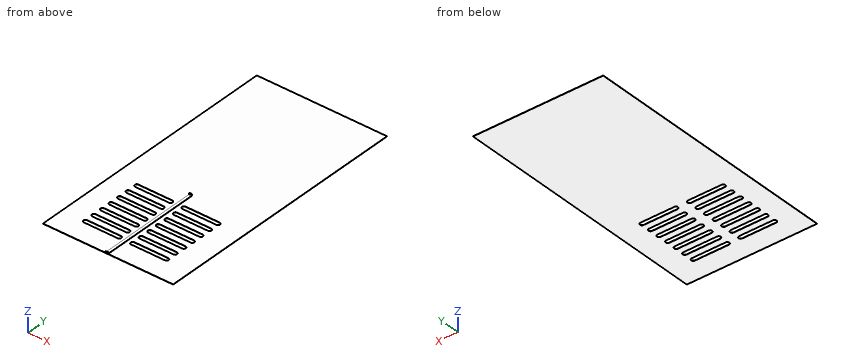
```python
from build123d import *

# Parameters (mm, degrees)
SKETCH1_W           = 500
SKETCH1_H           = 1000
BOSS_EXTRUDE1_DEPTH = 0.8
SKETCH4_W           = 10.782807929
SKETCH4_H           = 393.4
BOSS_EXTRUDE3_DEPTH = 0.8
SKETCH6_W           = 10.782807929
SKETCH6_H           = 5
BOSS_EXTRUDE4_DEPTH = 0.8
SKETCH7_W           = 10.782807929
SKETCH7_H           = 5
BOSS_EXTRUDE5_DEPTH = 0.8


with BuildPart() as part:
    # Sketch1 → Boss-Extrude1 (new body)
    with BuildSketch(Plane.XY):
        with Locations((250, 500)):
            Rectangle(SKETCH1_W, SKETCH1_H)
        with BuildLine():
            Line((89.759227751, 336.925516305), (219.774729178, 336.925516305))
            ThreePointArc((219.774729178, 336.925516305), (227.515924038, 329.184321446), (219.774729178, 321.443126586))
            Line((219.774729178, 321.443126586), (89.759227751, 321.443126586))
            ThreePointArc((89.759227751, 321.443126586), (82.018032891, 329.184321446), (89.759227751, 336.925516305))
        make_face(mode=Mode.SUBTRACT)
        with BuildLine():
            Line((271.405433716, 336.925516305), (401.890305185, 336.925516305))
            ThreePointArc((401.890305185, 336.925516305), (409.631500044, 329.184321446), (401.890305185, 321.443126586))
            Line((401.890305185, 321.443126586), (271.405433716, 321.443126586))
            ThreePointArc((271.405433716, 321.443126586), (263.664238856, 329.184321446), (271.405433716, 336.925516305))
        make_face(mode=Mode.SUBTRACT)
        with BuildLine():
            Line((271.405433716, 281.443126586), (401.890305185, 281.443126586))
            ThreePointArc((401.890305185, 281.443126586), (409.631500044, 289.184321446), (401.890305185, 296.925516305))
            Line((401.890305185, 296.925516305), (271.405433716, 296.925516305))
            ThreePointArc((271.405433716, 296.925516305), (263.664238856, 289.184321446), (271.405433716, 281.443126586))
        make_face(mode=Mode.SUBTRACT)
        with BuildLine():
            Line((89.759227751, 281.443126586), (219.774729178, 281.443126586))
            ThreePointArc((219.774729178, 281.443126586), (227.515924038, 289.184321446), (219.774729178, 296.925516305))
            Line((219.774729178, 296.925516305), (89.759227751, 296.925516305))
            ThreePointArc((89.759227751, 296.925516305), (82.018032891, 289.184321446), (89.759227751, 281.443126586))
        make_face(mode=Mode.SUBTRACT)
        with BuildLine():
            Line((271.405433716, 256.925516305), (401.890305185, 256.925516305))
            ThreePointArc((401.890305185, 256.925516305), (409.631500044, 249.184321446), (401.890305185, 241.443126586))
            Line((401.890305185, 241.443126586), (271.405433716, 241.443126586))
            ThreePointArc((271.405433716, 241.443126586), (263.664238856, 249.184321446), (271.405433716, 256.925516305))
        make_face(mode=Mode.SUBTRACT)
        with BuildLine():
            Line((271.405433716, 201.443126586), (401.890305185, 201.443126586))
            ThreePointArc((401.890305185, 201.443126586), (409.631500044, 209.184321446), (401.890305185, 216.925516305))
            Line((401.890305185, 216.925516305), (271.405433716, 216.925516305))
            ThreePointArc((271.405433716, 216.925516305), (263.664238856, 209.184321446), (271.405433716, 201.443126586))
        make_face(mode=Mode.SUBTRACT)
        with BuildLine():
            Line((89.759227751, 256.925516305), (219.774729178, 256.925516305))
            ThreePointArc((219.774729178, 256.925516305), (227.515924038, 249.184321446), (219.774729178, 241.443126586))
            Line((219.774729178, 241.443126586), (89.759227751, 241.443126586))
            ThreePointArc((89.759227751, 241.443126586), (82.018032891, 249.184321446), (89.759227751, 256.925516305))
        make_face(mode=Mode.SUBTRACT)
        with BuildLine():
            Line((89.759227751, 201.443126586), (219.774729178, 201.443126586))
            ThreePointArc((219.774729178, 201.443126586), (227.515924038, 209.184321446), (219.774729178, 216.925516305))
            Line((219.774729178, 216.925516305), (89.759227751, 216.925516305))
            ThreePointArc((89.759227751, 216.925516305), (82.018032891, 209.184321446), (89.759227751, 201.443126586))
        make_face(mode=Mode.SUBTRACT)
        with BuildLine():
            Line((271.405433716, 176.925516305), (401.890305185, 176.925516305))
            ThreePointArc((401.890305185, 176.925516305), (409.631500044, 169.184321446), (401.890305185, 161.443126586))
            Line((401.890305185, 161.443126586), (271.405433716, 161.443126586))
            ThreePointArc((271.405433716, 161.443126586), (263.664238856, 169.184321446), (271.405433716, 176.925516305))
        make_face(mode=Mode.SUBTRACT)
        with BuildLine():
            Line((89.759227751, 176.925516305), (219.774729178, 176.925516305))
            ThreePointArc((219.774729178, 176.925516305), (227.515924038, 169.184321446), (219.774729178, 161.443126586))
            Line((219.774729178, 161.443126586), (89.759227751, 161.443126586))
            ThreePointArc((89.759227751, 161.443126586), (82.018032891, 169.184321446), (89.759227751, 176.925516305))
        make_face(mode=Mode.SUBTRACT)
        with BuildLine():
            Line((89.759227751, 121.443126586), (219.774729178, 121.443126586))
            ThreePointArc((219.774729178, 121.443126586), (227.515924038, 129.184321446), (219.774729178, 136.925516305))
            Line((219.774729178, 136.925516305), (89.759227751, 136.925516305))
            ThreePointArc((89.759227751, 136.925516305), (82.018032891, 129.184321446), (89.759227751, 121.443126586))
        make_face(mode=Mode.SUBTRACT)
        with BuildLine():
            Line((271.405433716, 121.443126586), (401.890305185, 121.443126586))
            ThreePointArc((401.890305185, 121.443126586), (409.631500044, 129.184321446), (401.890305185, 136.925516305))
            Line((401.890305185, 136.925516305), (271.405433716, 136.925516305))
            ThreePointArc((271.405433716, 136.925516305), (263.664238856, 129.184321446), (271.405433716, 121.443126586))
        make_face(mode=Mode.SUBTRACT)
        with BuildLine():
            Line((271.405433716, 96.925516305), (401.890305185, 96.925516305))
            ThreePointArc((401.890305185, 96.925516305), (409.631500044, 89.184321446), (401.890305185, 81.443126586))
            Line((401.890305185, 81.443126586), (271.405433716, 81.443126586))
            ThreePointArc((271.405433716, 81.443126586), (263.664238856, 89.184321446), (271.405433716, 96.925516305))
        make_face(mode=Mode.SUBTRACT)
        with BuildLine():
            Line((89.759227751, 96.925516305), (219.774729178, 96.925516305))
            ThreePointArc((219.774729178, 96.925516305), (227.515924038, 89.184321446), (219.774729178, 81.443126586))
            Line((219.774729178, 81.443126586), (89.759227751, 81.443126586))
            ThreePointArc((89.759227751, 81.443126586), (82.018032891, 89.184321446), (89.759227751, 96.925516305))
        make_face(mode=Mode.SUBTRACT)
    extrude(amount=BOSS_EXTRUDE1_DEPTH)

    # Sketch4 → Boss-Extrude3 (add)
    with BuildSketch(Plane.XY.offset(0.8)):
        with Locations((244.608596036, 196.7)):
            Rectangle(SKETCH4_W, SKETCH4_H)
    extrude(amount=BOSS_EXTRUDE3_DEPTH)

    # Sketch6 → Boss-Extrude4 (add)
    with BuildSketch(Plane(origin=(0, 393.4, 0), x_dir=(1, 0, 0), z_dir=(0, 1, 0))):
        with Locations((244.608596036, -4.1)):
            Rectangle(SKETCH6_W, SKETCH6_H)
    extrude(amount=-BOSS_EXTRUDE4_DEPTH)

    # Sketch7 → Boss-Extrude5 (add)
    with BuildSketch(Plane(origin=(0, 0, 0), x_dir=(-1, 0, 0), z_dir=(0, -1, 0))):
        with Locations((-244.608596036, -4.1)):
            Rectangle(SKETCH7_W, SKETCH7_H)
    extrude(amount=-BOSS_EXTRUDE5_DEPTH)


solid = part.part
```
Could you check a few things on this model? Use its own coordinates, in mm. Coordinates: 2 decimals unless noted, no trailing zeros. Write each loop counter-clockwise with the first axis right and the second up, starting at its lowest first coordinate (ties: lowest second). Pieces come first, ordered by that corner, then holes. Notation, with made-up numbers: (-12, 87) -> (45, 87) arc R16 ccw to (45, 95) -> close; hole circle Ø4 at (69.5, -5.5). An arc over 180 degrees is marked (long way). One line per question, with ' | ' between items. Start each with the question number.
1. Will these pins go through, and if not, where does the flat tip stop? P1, Ø4, axis at x = 77, y = 395, coming from the +Z side; P2, Ø3, axis at y = 194, z = 4, coming from the -X side; P3, Ø5.5, axis at x = 245, y = 243.5, coming from the +Z side.
2. If we section it at A-A (x = 140): Count the separate pieces of the cut face and the enclosed holes in it, and give its area (3 significant figures).
3. If we section it at C-C (y = 61): Please give me the cut outline in (x, z).
4. If we section it at D-D (x = 441): Please give me the cut outline in (y, z).
5. Please list where these lines run through material, in increasing order: line 1 along Y through (x, z) = (242, 1.75); line 2 along X through (y, z) = (255, 0.75); line 3 along Z through (x, y) = (45, 157).
6. If we section it at B-B (z = 3.5): Please give me the cut outline in (x, y), and give its area (3 significant figures).
Return value:
1) P1: stops at z = 0.8 | P2: passes through | P3: stops at z = 1.6
2) separate pieces: 8 | enclosed holes: 0 | area: 713 mm²
3) outline: (0, 0) -> (500, 0) -> (500, 0.8) -> (250, 0.8) -> (250, 1.6) -> (239.22, 1.6) -> (239.22, 0.8) -> (0, 0.8) -> close
4) outline: (0, 0) -> (1000, 0) -> (1000, 0.8) -> (0, 0.8) -> close
5) line 1: y = 0 to 0.8, 392.6 to 393.4 | line 2: x = 0 to 84.65, 224.88 to 266.3, 407 to 500 | line 3: z = 0 to 0.8
6) outline: (239.22, 0) -> (250, 0) -> (250, 0.8) -> (239.22, 0.8) -> close; (239.22, 392.6) -> (250, 392.6) -> (250, 393.4) -> (239.22, 393.4) -> close | area: 17.3 mm²
